Design review of the part shown in the three views and the two pictorial views. Dimensions are in mm from the part's minimum x, y and z. A direction names the side the tool comes from. Give positions to 0.01 mm unless a question says otherwise; leave off trailing zeros. Write each loop counter-clockwise with the first axis right and the second up, starting at its lowest first coordinate (ties: lowest second). Pieces come first, ordered by that corner, then holes.
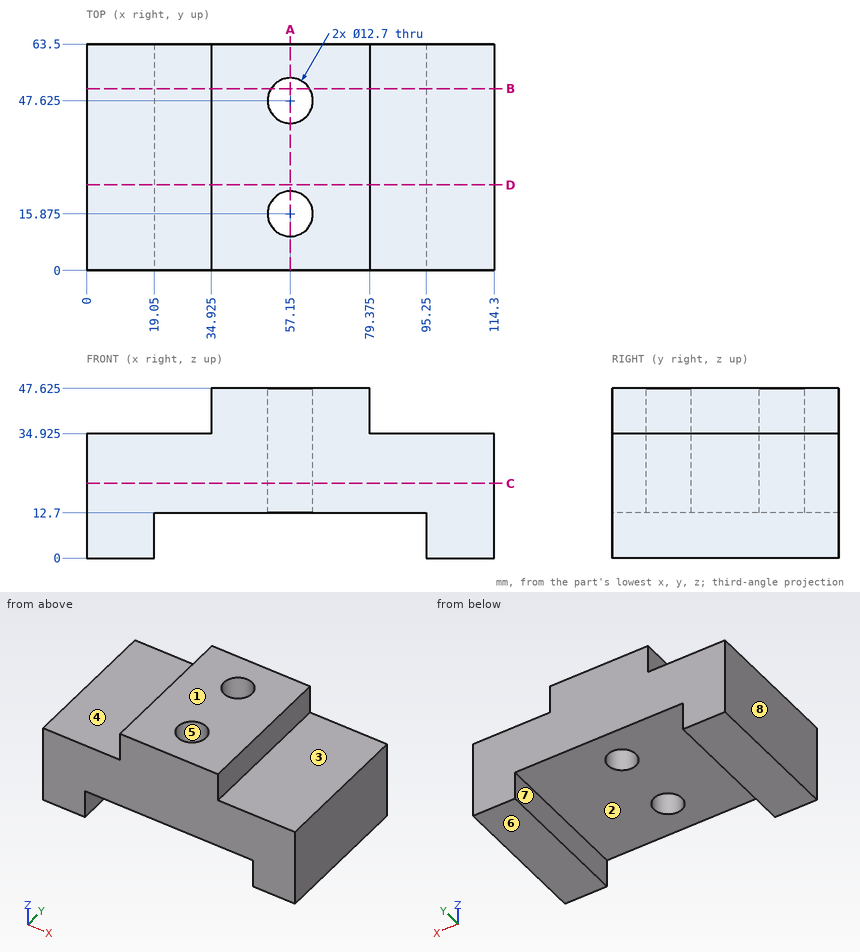
(1) Consider section B-B, the plane y = 51. Give the boundary of the cut face in (x, z) (3 decimals).
Resolved:
outline: (0, 0) - (19.05, 0) - (19.05, 12.7) - (51.771, 12.7) - (51.771, 47.625) - (34.925, 47.625) - (34.925, 34.925) - (0, 34.925) - close; (62.529, 12.7) - (95.25, 12.7) - (95.25, 0) - (114.3, 0) - (114.3, 34.925) - (79.375, 34.925) - (79.375, 47.625) - (62.529, 47.625) - close
(2) Tool access review of the marked faces 1, 2, 3 and 4: name each direction out of +Z, -Z, +X, -X, +Y, -Y from which nothing blocks a thin tool from reaching the whole face with its end or side.
Resolved:
face 1: +Z, +X, -X, +Y, -Y
face 2: -Z, +Y, -Y
face 3: +Z, +X, +Y, -Y
face 4: +Z, -X, +Y, -Y
(3) Clearance check with flat-ended pins moving along their axes: P1, Ø14.5, axis at x = 57.15, y = 47.625, coming from the -Z side; P2, Ø6.5, axis at y = 19.5, z = 40, coming from the +X side (3 decimals). State where each tip first meets the part, or that it passes through.
Resolved:
P1: stops at z = 12.7
P2: stops at x = 79.375
(4) Consider section A-A, the plane x = 57.15. Give the boundary of the cut face in (y, z) (3 decimals).
Resolved:
outline: (0, 12.7) - (9.525, 12.7) - (9.525, 47.625) - (0, 47.625) - close; (22.225, 12.7) - (41.275, 12.7) - (41.275, 47.625) - (22.225, 47.625) - close; (53.975, 12.7) - (63.5, 12.7) - (63.5, 47.625) - (53.975, 47.625) - close
(5) Mouldability with a two-part tool opening along X and no side actions: class the marked faces 5, 6, 7 and 8 as pulls with the +X half, pulls with the -X half, needs draft (parallel to the pull), parting line crosses it, or undercut.
Resolved:
face 5: undercut
face 6: needs draft
face 7: undercut
face 8: pulls with the -X half
(6) Consider section C-C, the plane z = 21. Give the boundary of the cut face in (x, y) (3 decimals).
Resolved:
outline: (0, 0) - (114.3, 0) - (114.3, 63.5) - (0, 63.5) - close; hole circle Ø12.7 at (57.15, 15.875); hole circle Ø12.7 at (57.15, 47.625)
(7) Consider section D-D, the plane y = 24. Give the boundary of the cut face in (x, z) (3 decimals).
Resolved:
outline: (0, 0) - (19.05, 0) - (19.05, 12.7) - (95.25, 12.7) - (95.25, 0) - (114.3, 0) - (114.3, 34.925) - (79.375, 34.925) - (79.375, 47.625) - (34.925, 47.625) - (34.925, 34.925) - (0, 34.925) - close
(8) To check wall thickness, follow L1, parallel to Y at x = 57, z = 33; L2, parallel to X at y = 51, z = 5.5; L3, parallel to X at y = 15.5, z = 14.5. State the ranges of each line that lie inside material, in increasing order.
Resolved:
L1: y = 0 to 9.53, 22.22 to 41.28, 53.97 to 63.5
L2: x = 0 to 19.05, 95.25 to 114.3
L3: x = 0 to 50.81, 63.49 to 114.3
